from build123d import *

# Parameters (mm, degrees)
ESQUISSE1_R        = 1.5
BOSS_EXTRU_1_DEPTH = 2.5


with BuildPart() as part:
    # Esquisse1 → Boss.-Extru.1 (new body)
    with BuildSketch(Plane(origin=(0, 0, 0), x_dir=(1, 0, 0), z_dir=(0, 1, 0))):
        Polygon((-30, -5), (-10, -5), (-10, -35), (10, -35), (10, -5), (30, -5), (30, 5), (-30, 5), align=None)
        with Locations((-25, 0)):
            Circle(ESQUISSE1_R, mode=Mode.SUBTRACT)
        with Locations((25, 0)):
            Circle(ESQUISSE1_R, mode=Mode.SUBTRACT)
        with Locations((-5, 0)):
            Circle(ESQUISSE1_R, mode=Mode.SUBTRACT)
        with Locations((5, 0)):
            Circle(ESQUISSE1_R, mode=Mode.SUBTRACT)
        with Locations((-5, -30)):
            Circle(ESQUISSE1_R, mode=Mode.SUBTRACT)
        with Locations((5, -30)):
            Circle(ESQUISSE1_R, mode=Mode.SUBTRACT)
        with Locations((0, -30)):
            Circle(ESQUISSE1_R, mode=Mode.SUBTRACT)
        with Locations((0, -20)):
            Circle(ESQUISSE1_R, mode=Mode.SUBTRACT)
        with Locations((0, -10)):
            Circle(ESQUISSE1_R, mode=Mode.SUBTRACT)
    extrude(amount=BOSS_EXTRU_1_DEPTH)


solid = part.part
Source: CAD feature listing. Evaluate the final solid. Frame: model axes, mm. A direction names the side the tool comes from. Give positions to 0.01 mm unless a question says otherwise; leave off trailing zeros. Write each loop counter-clockwise with the first axis right and the second up, starting at its lowest first coordinate (ties: lowest second). Pieces come first, ordered by that corner, then holes. Notation, with made-up numbers: (17.5, 58.5) - (53.5, 58.5) arc R32 ccw to (53.5, 84.5) - close; hole circle Ø10 at (66.5, 4). An arc over 180 degrees is marked (long way). Write item = value, one per line. Start each with the question number.
Q1. Cut plane C-C, the plane y = 0.7. Give the number of separate pieces and of enclosed holes in the cut face, then the cut area to 3 significant figures.
Q2. Pin query (flat end, axial travel): pin 1 Ø2.5 at (x, z) = (25, 0) entering from +Y; pin 2 Ø3.5 at (x, z) = (-5, 30) entering from -Y; pin 3 Ø1.2 at (x, y) = (-23.5, 1) entering from +Z; pin 4 Ø1.2 at (y, z) = (1.5, 17) entering from +X. Return the tip coordinate at first contact, or that it passes through.
Q3. Cut plane D-D, the plane z = 0. Return loops of the section in (x, y), then the cut area to 3 significant figures.
Q4. Reachability of faces 4 (the flat face through (-10, 1, 20)), 5 (the flat face through (0, 1, 35)), 6 (the flat face through (10, 1, 20)) from +Z, -Z, +X, -X, +Y, -Y: full face, straight path, thin tool, end or side. Return the list, or none.
Q5. Cut plane A-A, the plane z = 20. Return loops of the section in (x, y).
Q6. Material intervals for probe 1 along Z at (x, y) = (0, 0.9); probe 2 along X at (y, z) = (1.1, 30); probe 3 along Z at (x, y) = (5, 1.7), sorted ascending.
Q7. Cut plane B-B, the plane x = -25. Return loops of the section in (y, z), then the cut area to 3 significant figures.
Q8. Draft query along Z for faces 1 (the cylindrical face through (-0.325, 1.232, 11.464)), 2 (the flat face through (-30, 1, 0)), 3 (the flat face through (0, 1, -5)). Return one class per face: +Z half, -Z half, draft (parallel to the pull), parting line (faces both ways), or undercut.
Computed values:
q1.separate_pieces = 1
q1.enclosed_holes = 9
q1.area = 1,140 mm²
q2.pin_1 = through
q2.pin_2 = 0
q2.pin_3 = 5
q2.pin_4 = 10
q3.outline = (-30, 0) - (-26.5, 0) - (-26.5, 2.5) - (-30, 2.5) - close; (-23.5, 0) - (-6.5, 0) - (-6.5, 2.5) - (-23.5, 2.5) - close; (-3.5, 0) - (3.5, 0) - (3.5, 2.5) - (-3.5, 2.5) - close; (6.5, 0) - (23.5, 0) - (23.5, 2.5) - (6.5, 2.5) - close; (26.5, 0) - (30, 0) - (30, 2.5) - (26.5, 2.5) - close
q3.area = 120 mm²
q4.face_4 = +Z, -X, +Y, -Y
q4.face_5 = +Z, +X, -X, +Y, -Y
q4.face_6 = +Z, +X, +Y, -Y
q5.outline = (-10, 0) - (-1.5, 0) - (-1.5, 2.5) - (-10, 2.5) - close; (1.5, 0) - (10, 0) - (10, 2.5) - (1.5, 2.5) - close
q6.probe_1 = -5 to 8.5, 11.5 to 18.5, 21.5 to 28.5, 31.5 to 35
q6.probe_2 = -10 to -6.5, -3.5 to -1.5, 1.5 to 3.5, 6.5 to 10
q6.probe_3 = -5 to -1.5, 1.5 to 28.5, 31.5 to 35
q7.outline = (0, -5) - (2.5, -5) - (2.5, -1.5) - (0, -1.5) - close; (0, 1.5) - (2.5, 1.5) - (2.5, 5) - (0, 5) - close
q7.area = 17.5 mm²
q8.face_1 = undercut
q8.face_2 = draft
q8.face_3 = -Z half
